from build123d import *

# Parameters (mm, degrees)
SKETCH1_W           = 38
SKETCH1_H           = 22
BOSS_EXTRUDE1_DEPTH = 33
SKETCH2_W           = 35
SKETCH2_H           = 17
CUT_EXTRUDE1_DEPTH  = 28
SKETCH3_W           = 6
SKETCH3_H           = 17
BOSS_EXTRUDE2_DEPTH = 17.5
SKETCH4_W           = 42
SKETCH4_H           = 26
SKETCH4_W_2         = 38
SKETCH4_H_2         = 22
EXTRUDE_THIN2_DEPTH = 1.4
SKETCH5_R           = 1
CUT_EXTRUDE2_DEPTH  = 3
SKETCH6_R           = 1
CUT_EXTRUDE3_DEPTH  = 3
SKETCH7_W           = 9.4
SKETCH7_H           = 4.5
CUT_EXTRUDE4_DEPTH  = 10
SKETCH8_W           = 20
SKETCH8_H           = 10
CUT_EXTRUDE5_DEPTH  = 1.5
SKETCH9_R           = 3.7
SKETCH9_R_2         = 1
CUT_EXTRUDE6_DEPTH  = 1.7
FILLET1_R           = 4
BOSS_EXTRUDE3_START = -22
BOSS_EXTRUDE3_DEPTH = 22
FILLET2_R           = 3


with BuildPart() as part:
    # Sketch1 → Boss-Extrude1 (new body)
    with BuildSketch(Plane(origin=(0, 0, 0), x_dir=(1, 0, 0), z_dir=(0, 1, 0))):
        with Locations((8.6, -5.057142857)):
            Rectangle(SKETCH1_W, SKETCH1_H)
    extrude(amount=BOSS_EXTRUDE1_DEPTH)

    # Sketch2 → Cut-Extrude1 (cut)
    with BuildSketch(Plane(origin=(0, 33, 0), x_dir=(1, 0, 0), z_dir=(0, 1, 0))):
        with Locations((8.5, -3.957142857)):
            Rectangle(SKETCH2_W, SKETCH2_H)
    extrude(amount=-CUT_EXTRUDE1_DEPTH, mode=Mode.SUBTRACT)

    # Sketch3 → Boss-Extrude2 (add)
    with BuildSketch(Plane(origin=(0, 5, 0), x_dir=(1, 0, 0), z_dir=(0, 1, 0))):
        with Locations((-6, -3.957142857)):
            Rectangle(SKETCH3_W, SKETCH3_H)
        with Locations((23, -3.957142857)):
            Rectangle(SKETCH3_W, SKETCH3_H)
    extrude(amount=BOSS_EXTRUDE2_DEPTH)

    # Sketch4 → Extrude-Thin2 (add)
    with BuildSketch(Plane(origin=(0, 33, 0), x_dir=(1, 0, 0), z_dir=(0, 1, 0))):
        with Locations((8.6, -5.057142857)):
            Rectangle(SKETCH4_W, SKETCH4_H)
        with Locations((8.6, -5.057142857)):
            Rectangle(SKETCH4_W_2, SKETCH4_H_2, mode=Mode.SUBTRACT)
    extrude(amount=-EXTRUDE_THIN2_DEPTH)

    # Sketch5 → Cut-Extrude2 (cut)
    with BuildSketch(Plane(origin=(0, 22.5, 0), x_dir=(1, 0, 0), z_dir=(0, 1, 0))):
        with Locations(Location((-5.5, -3.892148731, 0), (0, 0, 270))):
            Circle(SKETCH5_R)
    extrude(amount=-CUT_EXTRUDE2_DEPTH, mode=Mode.SUBTRACT)

    # Sketch6 → Cut-Extrude3 (cut)
    with BuildSketch(Plane(origin=(0, 22.5, 0), x_dir=(1, 0, 0), z_dir=(0, 1, 0))):
        with Locations(Location((22.953148274, -4.115727136, 0), (0, 0, 270))):
            Circle(SKETCH6_R)
    extrude(amount=-CUT_EXTRUDE3_DEPTH, mode=Mode.SUBTRACT)

    # Sketch7 → Cut-Extrude4 (cut)
    with BuildSketch(Plane(origin=(-3, 0, 0), x_dir=(0, 0, -1), z_dir=(1, 0, 0))):
        with Locations((-3.757142857, 6.291369126)):
            Rectangle(SKETCH7_W, SKETCH7_H)
    extrude(amount=-CUT_EXTRUDE4_DEPTH, mode=Mode.SUBTRACT)

    # Sketch8 → Cut-Extrude5 (cut)
    with BuildSketch(Plane(origin=(0, 5, 0), x_dir=(1, 0, 0), z_dir=(0, 1, 0))):
        with Locations((8.592117784, -3.72787339)):
            Rectangle(SKETCH8_W, SKETCH8_H)
    extrude(amount=-CUT_EXTRUDE5_DEPTH, mode=Mode.SUBTRACT)

    # Sketch9 → Cut-Extrude6 (cut)
    with BuildSketch(Plane(origin=(0, 3.5, 0), x_dir=(1, 0, 0), z_dir=(0, 1, 0))):
        with Locations(Location((8.808284604, -3.634888569, 0), (0, 0, 270))):
            Circle(SKETCH9_R)
        with Locations(Location((1.608284604, -3.634888569, 0), (0, 0, 270))):
            Circle(SKETCH9_R_2)
        with Locations(Location((16.008284604, -3.634888569, 0), (0, 0, 270))):
            Circle(SKETCH9_R_2)
    extrude(amount=-CUT_EXTRUDE6_DEPTH, mode=Mode.SUBTRACT)

    # Fillet1
    fillet1_edges = [part.edges().sort_by_distance(p)[0] for p in [
        (-1.407882216, 4.25, 8.72787339),
        (-1.407882216, 4.25, -1.27212661),
        (18.592117784, 4.25, -1.27212661),
        (18.592117784, 4.25, 8.72787339),
    ]]
    fillet(fillet1_edges, radius=FILLET1_R)

    # Sketch10 → Boss-Extrude3 (add)
    with BuildSketch(Plane.XY.offset(16.057142857).offset(BOSS_EXTRUDE3_START)):
        Polygon((27.6, 31.6), (29.607360767, 31.6), (27.6, 27.732810295), align=None)
    extrude(amount=BOSS_EXTRUDE3_DEPTH)

    # Fillet2
    fillet2_edges = [part.edges().sort_by_distance(p)[0] for p in [
        (-3, 8.541369126, 3.757142857),
    ]]
    fillet(fillet2_edges, radius=FILLET2_R)


solid = part.part
Build history of the part. All positions in model axes, mm. A direction names the side the tool comes from. Give positions to 0.01 mm unless a question says otherwise; leave off trailing zeros. Order: outer loops, then holes, each group sorted by start corner. A loop starts at its lowest first (then second) coordinate and runs counter-clockwise, first axis right, second up. Notation, with made-up numbers: M 48,61.25 L 62,61.25 A26 ccw 62,75.25 Z; hole C -27.75,68.25 d2. An arc over 180 degrees is marked long. Put each result on its own line as item: value.
Item 1: Cut at B-B on x = -8. Write the cut outline in (y, z), then the cut area to 3 significant figures.
Results are:
outline: M 0,-5.94 L 31.6,-5.94 L 31.6,-7.94 L 33,-7.94 L 33,-4.54 L 22.5,-4.54 L 22.5,12.46 L 33,12.46 L 33,18.06 L 31.6,18.06 L 31.6,16.06 L 0,16.06 Z; hole M 4.04,-0.94 L 8.54,-0.94 L 8.54,8.46 L 4.04,8.46 Z
area: 511 mm2
Item 2: Pull direction X, two halves, no side cores. Call faces 1 (the face through (-7, 4.041, 4)), 2 (the face through (23, 19.5, 4)), 3 (the face through (-3, 4.5, 3.8)): +X half, -X half, draft (parallel to the pull), parting line (faces both ways), or undercut.
Results are:
face 1: draft
face 2: undercut
face 3: -X half
Item 3: Cut at D-D on x = 4.5. Write the cut outline in (y, z).
Results are:
outline: M 0,-5.94 L 31.6,-5.94 L 31.6,-7.94 L 33,-7.94 L 33,-4.54 L 5,-4.54 L 5,-1.27 L 3.5,-1.27 L 3.5,8.73 L 5,8.73 L 5,12.46 L 33,12.46 L 33,18.06 L 31.6,18.06 L 31.6,16.06 L 0,16.06 Z
Item 4: Cut at A-A on y = 25. Write the cut outline in (x, z), then the cut area to 3 significant figures.
Results are:
outline: M -10.4,-5.94 L 27.6,-5.94 L 27.6,16.06 L -10.4,16.06 Z; hole M -9,-4.54 L 26,-4.54 L 26,12.46 L -9,12.46 Z
area: 241 mm2
Item 5: Drop flat-ended pins along their axis: pin 1 Ø2.5 at (x, z) = (1.61, 3.63) entering from +Y; pin 2 Ø6 at (x, z) = (-5.5, 5) entering from +Y; pin 3 Ø3 at (x, y) = (1.5, 7.5) entering from +Z. Give the stop position or say it passes through.
Results are:
pin 1: y = 3.5
pin 2: y = 22.5
pin 3: z = 16.06
Item 6: Wall check: probe 1 along Z at (x, y) = (8.5, 27); probe 2 along X at (y, z) = (6, 9.25); probe 3 along Z at (x, y) = (-4, 9). Give the ranges that are in metal, low to high.
Results are:
probe 1: -5.94 to -4.54, 12.46 to 16.06
probe 2: -10.4 to -3, 20 to 27.6
probe 3: -5.94 to -0.94, 8.46 to 16.06
Item 7: Which spindle directions (+Z, -Z, +X, -X, +Y, -Y) get a long thin tool onto all of the face, cutting with end or side? Do faces 4 (the face through (11, 3.5, 0)), 5 (the face through (-10.4, 16, 5)). Say none if no direction does.
Results are:
face 4: +Y
face 5: +Z, -Z, -X, -Y
